Build history of the part. All positions in model axes, mm. A direction names the side the tool comes from. Give positions to 0.01 mm unless a question says otherwise; leave off trailing zeros. Write each loop counter-clockwise with the first axis right and the second up, starting at its lowest first coordinate (ties: lowest second). Pieces come first, ordered by that corner, then holes. Notation, with made-up numbers: (34.5, 52.25) -> (79.5, 52.25) arc R33 cw to (79.5, 83.25) -> close; hole circle Ø11 at (60, -33). An arc over 180 degrees is marked (long way). One line per question, with ' | ' between items. Start each with the question number.
(1) Band-saw the part on C-C, the plane y = 2. Give the cut face in (x, z).
(2) Band-saw the part on A-A, the plane x = 15. Give the cut face in (y, z), and give its area (3 significant figures).
(3) Pull direction Z, two halves, no side cores. Call faces 4 (the flat face through (0.5, 2.5, -29.5)), 5 (the flat face through (47.5, 2.5, -0.5)), 6 (the cylindrical face through (5.971, 1.75, -27.686)): released by +Z, released by -Z, zero draft, split by the parting line, or undercut.
(4) Band-saw the part on B-B, the plane z = -26. Give the cut face in (x, y).
(5) Pin check, flat tips, straight feed: P1, Ø3, axis at x = 33, z = 4, coming from the +Y side; P2, Ø1.5, axis at x = 39.5, y = 4, coming from the +Z side. Stop position of each tip, or through.
(6) Band-saw the part on D-D, the plane x = 42.25. Give the cut face in (y, z), and give its area (3 significant figures).
(7) Drill centre lines: probe 1 along X at (y, z) = (0.85, -26); probe 2 along X at (y, z) = (3.8, -26); probe 3 along Z at (x, y) = (42.25, 2.45). Where is each one in solid material? Low to high. Write a range as from..to.
(8) Tool access for faces 1 (the flat face through (47.5, 2.5, -29.5)), 2 (the flat face through (38, 2, 3)), 3 (the flat face through (6, 2, 0)): list every direction of +Z, -Z, +X, -X, +Y, -Y with a clear straight run to the whole face (end or side of a thin tool).
from build123d import *

# Parameters (mm, degrees)
BOSS_EXTRUDE1_DEPTH                                 = 5
CSK_FOR_M3_FLAT_COUNTERSUNK_HEAD_SCREW1_D           = 3.4
CSK_FOR_M3_FLAT_COUNTERSUNK_HEAD_SCREW1_CSINK_D     = 6.3
CSK_FOR_M3_FLAT_COUNTERSUNK_HEAD_SCREW1_CSINK_ANGLE = 90
CHAMFER1_SIZE                                       = 1


with BuildPart() as part:
    # Sketch1 → Boss-Extrude1 (new body)
    with BuildSketch(Plane(origin=(0, 0, 0), x_dir=(1, 0, 0), z_dir=(0, 1, 0))):
        Polygon((0, 0), (0, 30), (48, 30), (48, 0), (38, 0), (38, -8), (10, -8), (10, 0), align=None)
    extrude(amount=BOSS_EXTRUDE1_DEPTH)

    # CSK for M3 Flat Countersunk Head Screw1 (through all)
    with Locations(Plane(origin=(0, 5, 0), x_dir=(1, 0, 0), z_dir=(0, 1, 0))):
        with Locations((5.75, 26), (42.25, 26), (15, -4), (33, -4)):
            CounterSinkHole(CSK_FOR_M3_FLAT_COUNTERSUNK_HEAD_SCREW1_D / 2, CSK_FOR_M3_FLAT_COUNTERSUNK_HEAD_SCREW1_CSINK_D / 2, counter_sink_angle=CSK_FOR_M3_FLAT_COUNTERSUNK_HEAD_SCREW1_CSINK_ANGLE)

    # Chamfer1
    chamfer1_edges = [part.edges().sort_by_distance(p)[0] for p in [
        (0, 2.5, 0),
        (0, 2.5, -30),
        (48, 2.5, -30),
        (48, 2.5, 0),
        (38, 2.5, 8),
        (10, 2.5, 8),
    ]]
    chamfer(chamfer1_edges, length=CHAMFER1_SIZE)


solid = part.part
Results:
1) outline: (0, -29) -> (1, -30) -> (47, -30) -> (48, -29) -> (48, -1) -> (47, 0) -> (38, 0) -> (38, 7) -> (37, 8) -> (11, 8) -> (10, 7) -> (10, 0) -> (1, 0) -> (0, -1) -> close; hole circle Ø3.4 at (5.75, -26); hole circle Ø3.4 at (15, 4); hole circle Ø3.4 at (33, 4); hole circle Ø3.4 at (42.25, -26)
2) outline: (0, -30) -> (5, -30) -> (5, 0.85) -> (3.55, 2.3) -> (0, 2.3) -> close; (0, 5.7) -> (3.55, 5.7) -> (5, 7.15) -> (5, 8) -> (0, 8) -> close | area: 171 mm²
3) face 4: released by -Z | face 5: released by +Z | face 6: undercut
4) outline: (0, 0) -> (4.05, 0) -> (4.05, 3.55) -> (2.6, 5) -> (0, 5) -> close; (7.45, 0) -> (40.55, 0) -> (40.55, 3.55) -> (39.1, 5) -> (8.9, 5) -> (7.45, 3.55) -> close; (43.95, 0) -> (48, 0) -> (48, 5) -> (45.4, 5) -> (43.95, 3.55) -> close
5) P1: passes through | P2: stops at z = 0
6) outline: (0, -30) -> (5, -30) -> (5, -29.15) -> (3.55, -27.7) -> (0, -27.7) -> close; (0, -24.3) -> (3.55, -24.3) -> (5, -22.85) -> (5, 0) -> (0, 0) -> close | area: 131 mm²
7) probe 1: x = 0..4.05, 7.45..40.55, 43.95..48 | probe 2: x = 0..3.8, 7.7..40.3, 44.2..48 | probe 3: z = -30..-27.7, -24.3..0
8) face 1: -Z, +X, +Y, -Y | face 2: +Z, +X, +Y, -Y | face 3: +Z, -X, +Y, -Y
